Here's how the part is built. I have some questions about the finished solid (model axes, mm). A direction names the side the tool comes from. Coordinates: 2 decimals unless noted, no trailing zeros. Write each loop counter-clockwise with the first axis right and the second up, starting at its lowest first coordinate (ties: lowest second). Pieces come first, ordered by that corner, then holes.
Item 1: For faces 1 (the face through (36.49, 10.504, -3.969)), 2 (the face through (-36.49, 10.136, 0.217)), 3 (the face through (-34.925, 11, -2)), which set-ups out of +Z, -Z, +X, -X, +Y, -Y let a thin tool reach every point of the face, with its end or its side?
Item 2: We'd pull the mould along Y, two halves only. Please class faces 4 (the face through (-38.1, 9, 0)), 5 (the face through (-0.2, 19.05, -8.3)), 6 (the face through (36.49, 10.136, 2.958)): +Y half, -Y half, draft (parallel to the pull), parting line (faces both ways), or undercut.
Item 3: If we section it at A-A (y = 14): Please give me the cut outline in (x, z) (1 decimal).
Item 4: If I drill on line 1 (Z direction, x = -4, y = 18); line 2 (X direction, y = 14.25, z = -7) (3 decimals); line 3 (Y direction, x = -37.2, z = 0), over which ranges is the centre line in solid material (lowest first)?
Item 5: I'm going to push a flat-ended pin straight in: pin 1 Ø1.5 at (x, z) = (30, -6) entering from +Y (3 decimals). Where does the tip first touch, or does it pass through?
Item 6: If we section it at D-D (z = -5.5): Please give me the cut outline in (x, y) (3 decimals), then the cut area to 3 significant figures.
from build123d import *

# Parameters (mm, degrees)
SKETCH1_W           = 76.2
SKETCH1_H           = 22.225
BOSS_EXTRUDE1_DEPTH = 3.175
SKETCH2_W           = 3.175
SKETCH2_H           = 15.875
BOSS_EXTRUDE2_DEPTH = 15.875
SKETCH3_R           = 1
CUT_EXTRUDE1_DEPTH  = 4.175
SKETCH4_R           = 1
CUT_EXTRUDE2_DEPTH  = 4.175


with BuildPart() as part:
    # Sketch1 → Boss-Extrude1 (new body)
    with BuildSketch(Plane(origin=(0, 0, 0), x_dir=(1, 0, 0), z_dir=(0, 1, 0))):
        Rectangle(SKETCH1_W, SKETCH1_H)
    extrude(amount=BOSS_EXTRUDE1_DEPTH)

    # Sketch2 → Boss-Extrude2 (add)
    with BuildSketch(Plane(origin=(0, 3.175, 0), x_dir=(1, 0, 0), z_dir=(0, 1, 0))):
        Polygon((38.1, 11.1125), (-38.1, 11.1125), (-38.1, 7.9375), (-34.925, 7.9375), (34.925, 7.9375), (38.1, 7.9375), align=None)
        with Locations((-36.5125, 0)):
            Rectangle(SKETCH2_W, SKETCH2_H)
        Polygon((-34.925, -7.9375), (-38.1, -7.9375), (-38.1, -11.1125), (38.1, -11.1125), (38.1, -7.9375), (34.925, -7.9375), align=None)
        with Locations((36.5125, 0)):
            Rectangle(SKETCH2_W, SKETCH2_H)
    extrude(amount=BOSS_EXTRUDE2_DEPTH)

    # Sketch3 → Cut-Extrude1 (cut, through all)
    with BuildSketch(Plane.ZY.offset(-34.925)):
        with Locations((3.175, 11.1125)):
            Circle(SKETCH3_R)
        with Locations((-3.175, 11.1125)):
            Circle(SKETCH3_R)
    extrude(amount=-CUT_EXTRUDE1_DEPTH, mode=Mode.SUBTRACT)

    # Sketch4 → Cut-Extrude2 (cut, through all)
    with BuildSketch(Plane(origin=(-34.925, 0, 0), x_dir=(0, 0, -1), z_dir=(1, 0, 0))):
        with Locations((0, 11.1125)):
            Circle(SKETCH4_R)
    extrude(amount=-CUT_EXTRUDE2_DEPTH, mode=Mode.SUBTRACT)


solid = part.part
Answer list:
1. face 1: +X
1. face 2: -X
1. face 3: +Y
2. face 4: draft
2. face 5: +Y half
2. face 6: undercut
3. outline: (-38.1, -11.1) - (38.1, -11.1) - (38.1, 11.1) - (-38.1, 11.1) - close; hole (-34.9, -7.9) - (34.9, -7.9) - (34.9, 7.9) - (-34.9, 7.9) - close
4. line 1: z = -11.11 to -7.94, 7.94 to 11.11
4. line 2: x = -38.1 to -34.925, 34.925 to 38.1
4. line 3: y = 0 to 10.11, 12.11 to 19.05
5. pin 1: stops at y = 3.175
6. outline: (-38.1, 0) - (38.1, 0) - (38.1, 19.05) - (34.925, 19.05) - (34.925, 3.175) - (-34.925, 3.175) - (-34.925, 19.05) - (-38.1, 19.05) - close
6. area: 343 mm2
